Answer from the drawing. Dimensions are ordinates in mm from the lowest x, y and z of the part. Give positions to 0.01 mm unless a question says otherwise; leave off trailing zeros. Order: outer loops, then holes, each group sorted by start corner. A loop starts at its lowest first (then second) coordinate and runs counter-clockwise, first axis right, second up. Notation, with made-up numbers: (49, 18) - (74, 18) arc R28 ccw to (74, 50) - close; hole circle Ø3 at (20.25, -20.5). An arc over 180 degrees is marked (long way). Use a Markdown table: item, result. Add a question column.
1) Find section B-B, the plane z = 3.5. Determine the outline of the cut face in (x, y), plus the area to 3 significant figures.
2) Straight lines are drawn through the part: line 1 (Y direction, x = 145, z = 3.05); line 2 (X direction, y = 256, z = 3.55); line 3 (Y direction, x = 152, z = 4.1). For each, find the intervals that lie inside material, in ascending order.
3) Find section D-D, the plane y = 42. Determine the outline of the cut face in (x, z), plus the area to 3 significant figures.
4) Flat-ended cylindrical pins translate along their axes: pin 1 (1 mm diameter, centred on x = 140.5, z = 3, fed in from +Y); pin 2 (3 mm diameter, centred on y = 368.5, z = 3.5, fed in from +X). Find the tip coordinate at first contact, or state that the pin passes through.
5) Find section C-C, the plane x = 145. Determine the outline of the cut face in (y, z).
6) Find section A-A, the plane y = 316. Determine the outline of the cut face in (x, z).
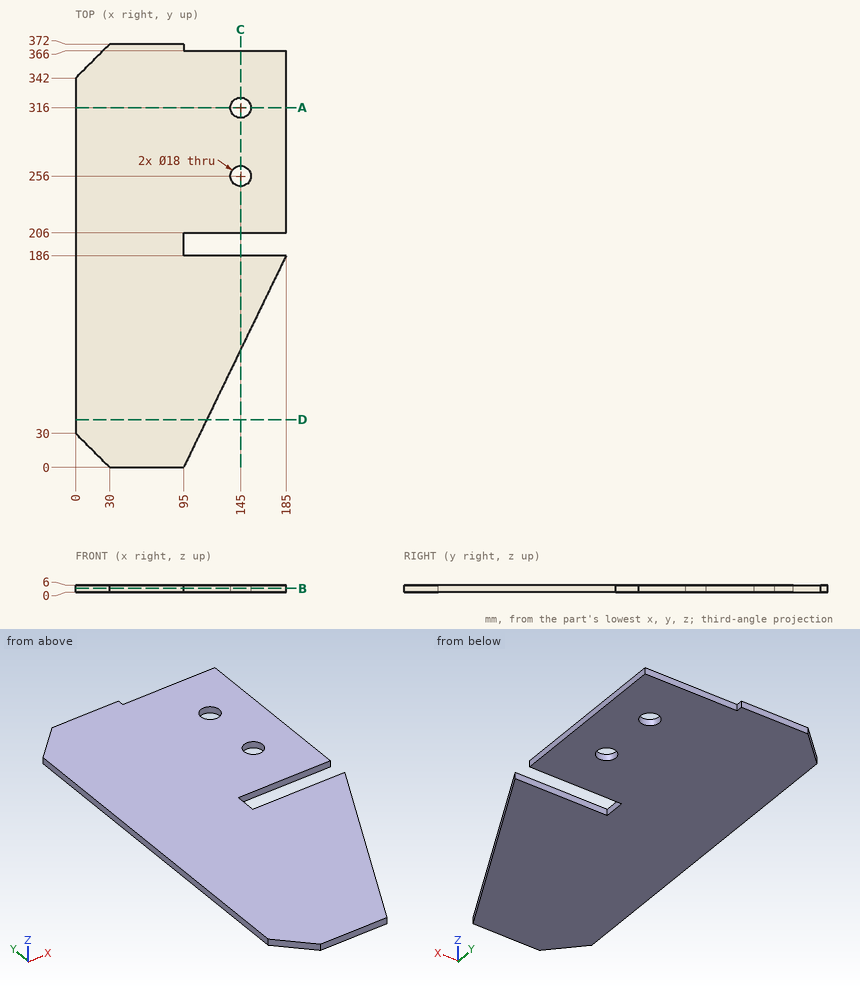
The answers:
| question | item | result |
|---|---|---|
| 1 | outline | (0, 30) - (30, 0) - (95, 0) - (185, 186) - (95, 186) - (95, 206) - (185, 206) - (185, 366) - (95, 366) - (95, 372) - (30, 372) - (0, 342) - close; hole circle Ø18 at (145, 256); hole circle Ø18 at (145, 316) |
| 1 | area | 56,700 mm2 |
| 2 | line 1 | 103.33 to 186, 206 to 247, 265 to 307, 325 to 366 |
| 2 | line 2 | 0 to 136, 154 to 185 |
| 2 | line 3 | 117.8 to 186, 206 to 250.34, 261.66 to 310.34, 321.66 to 366 |
| 3 | outline | (0, 0) - (115.32, 0) - (115.32, 6) - (0, 6) - close |
| 3 | area | 692 mm2 |
| 4 | pin 1 | y = 366 |
| 4 | pin 2 | x = 95 |
| 5 | outline | (103.33, 0) - (186, 0) - (186, 6) - (103.33, 6) - close; (206, 0) - (247, 0) - (247, 6) - (206, 6) - close; (265, 0) - (307, 0) - (307, 6) - (265, 6) - close; (325, 0) - (366, 0) - (366, 6) - (325, 6) - close |
| 6 | outline | (0, 0) - (136, 0) - (136, 6) - (0, 6) - close; (154, 0) - (185, 0) - (185, 6) - (154, 6) - close |
